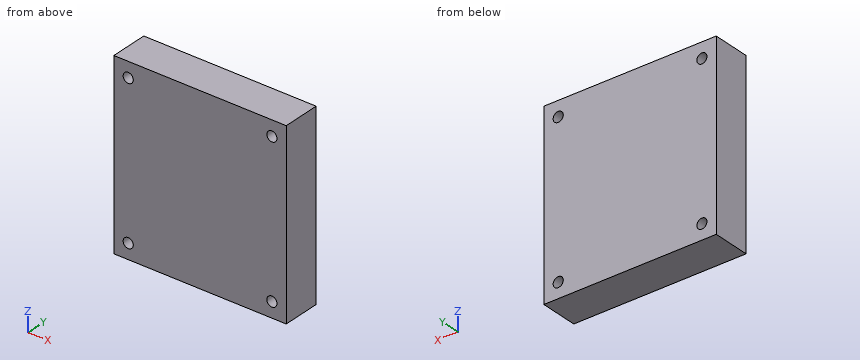
from build123d import *

# Parameters (mm, degrees)
SKETCH1_W                = 57.9
SKETCH1_H                = 61
EXTRUDE1_DEPTH           = 12.7
M3_CLEARANCE_HOLE1_D     = 3.4
M3_CLEARANCE_HOLE1_DEPTH = 12.7
M3_CLEARANCE_HOLE1_TIP   = 1.021463052


with BuildPart() as part:
    # Sketch1 → Extrude1 (new body)
    with BuildSketch(Plane(origin=(0, 0, 0), x_dir=(1, 0, 0), z_dir=(0, 1, 0))):
        Rectangle(SKETCH1_W, SKETCH1_H)
    extrude(amount=EXTRUDE1_DEPTH)

    # M3 Clearance Hole1
    with Locations(Plane(origin=(24.13, 0, -25.4), x_dir=(0, 0, -1), z_dir=(0, -1, 0))):
        with Locations((0, 0), (0, -48.26), (-50.8, -48.26), (-50.8, 0)):
            Hole(M3_CLEARANCE_HOLE1_D / 2, depth=M3_CLEARANCE_HOLE1_DEPTH)
            with Locations((0, 0, -(M3_CLEARANCE_HOLE1_DEPTH + M3_CLEARANCE_HOLE1_TIP / 2))):  # 118° drill point
                Cone(0, M3_CLEARANCE_HOLE1_D / 2, M3_CLEARANCE_HOLE1_TIP, mode=Mode.SUBTRACT)


solid = part.part
Check sheet for the modelled part. Datum: model origin and axes. Units: mm. Round coordinates to 2 decimals unless told otherwise and drop trailing zeros. Loops run counter-clockwise (first coordinate to the right, second up) from the corner with the lowest first, then second, coordinate; pieces in that order, holes last. Notation, with made-up numbers: (20.25, -19.75) - (34.25, -19.75) arc R18 cw to (34.25, 2.25) - close; hole circle Ø6 at (16.25, -28). An arc over 180 degrees is marked (long way). Answer as CSV lines item,"result". Start each with the question number.
Item 1: Section check B-B (x = 24.13). Record the boundary of the cut face in (y, z), and give its area (3 significant figures).
Item 2: Section check A-A (z = 25.4). Record the boundary of the cut face in (x, y), and give its area (3 significant figures).
Item 3: Depth check by flat-ended pin: P1, Ø1.5, axis at x = -10.5, z = 17, coming from the -Y side. Enter the tip coordinate at first touch or a pass-through.
Item 4: Scan lines: line 1 (X direction, y = 3, z = 25.4); line 2 (Z direction, x = -24.13, y = 9.75); line 3 (X direction, y = 9, z = 24). Record each from-to range of solid material in increasing order. Write a range as [from, to].
Report:
1,outline,"(0, -30.5) - (12.7, -30.5) - (12.7, -27.1) - (0, -27.1) - close; (0, -23.7) - (12.7, -23.7) - (12.7, 23.7) - (0, 23.7) - close; (0, 27.1) - (12.7, 27.1) - (12.7, 30.5) - (0, 30.5) - close"
1,area,"688 mm2"
2,outline,"(-28.95, 0) - (-25.83, 0) - (-25.83, 12.7) - (-28.95, 12.7) - close; (-22.43, 0) - (22.43, 0) - (22.43, 12.7) - (-22.43, 12.7) - close; (25.83, 0) - (28.95, 0) - (28.95, 12.7) - (25.83, 12.7) - close"
2,area,"649 mm2"
3,P1,"stops at y = 0"
4,line 1,"x = [-28.95, -25.83], [-22.43, 22.43], [25.83, 28.95]"
4,line 2,"z = [-30.5, -27.1], [-23.7, 23.7], [27.1, 30.5]"
4,line 3,"x = [-28.95, -25.09], [-23.17, 23.17], [25.09, 28.95]"
